```python
from build123d import *

# Parameters (mm, degrees)
SKETCH1_W           = 75
SKETCH1_H           = 90
BOSS_EXTRUDE1_DEPTH = 50
SKETCH2_W           = 75
SKETCH2_H           = 90
BOSS_EXTRUDE2_DEPTH = 10
BOSS_EXTRUDE2_TAPER = 45
SKETCH3_R           = 25
BOSS_EXTRUDE3_DEPTH = 10
SKETCH4_R           = 22.5
BOSS_EXTRUDE4_DEPTH = 30
SKETCH5_R           = 2.5
CUT_EXTRUDE1_DEPTH  = 5
CIRPATTERN1_COUNT   = 10
SKETCH6_W           = 20
SKETCH6_H           = 24
BOSS_EXTRUDE5_DEPTH = 100
SKETCH7_R           = 22.5
BOSS_EXTRUDE6_DEPTH = 10
SKETCH8_R           = 21.5
BOSS_EXTRUDE7_DEPTH = 20
SKETCH9_R           = 10
CUT_EXTRUDE2_DEPTH  = 10
FILLET1_RADIUS      = 45
FILLET1_LENGTH      = 75
SKETCH10_R          = 37.5
BOSS_EXTRUDE8_DEPTH = 10
BOSS_EXTRUDE8_TAPER = 45
SKETCH11_R          = 17.5
CUT_EXTRUDE3_DEPTH  = 20
FILLET4_R           = 1
FILLET5_R           = 1


with BuildPart() as part:
    # Sketch1 → Boss-Extrude1 (new, symmetric)
    with BuildSketch(Plane.XY):
        Rectangle(SKETCH1_W, SKETCH1_H)
    extrude(amount=BOSS_EXTRUDE1_DEPTH, both=True)

    # Sketch2 → Boss-Extrude2 (add)
    with BuildSketch(Plane(origin=(0, 0, -50), x_dir=(-1, 0, 0), z_dir=(0, 0, -1))):
        Rectangle(SKETCH2_W, SKETCH2_H)
    extrude(amount=BOSS_EXTRUDE2_DEPTH, taper=BOSS_EXTRUDE2_TAPER)

    # Sketch3 → Boss-Extrude3 (add)
    with BuildSketch(Plane(origin=(0, 0, -60), x_dir=(-1, 0, 0), z_dir=(0, 0, -1))):
        Circle(SKETCH3_R)
    extrude(amount=BOSS_EXTRUDE3_DEPTH)

    # Sketch4 → Boss-Extrude4 (add)
    with BuildSketch(Plane(origin=(0, 0, -70), x_dir=(-1, 0, 0), z_dir=(0, 0, -1))):
        Circle(SKETCH4_R)
    extrude(amount=BOSS_EXTRUDE4_DEPTH)

    # Sketch5 → Cut-Extrude1 (cut)
    with BuildSketch(Plane(origin=(0, 0, -100), x_dir=(-1, 0, 0), z_dir=(0, 0, -1))):
        with Locations((18, 0)):
            Circle(SKETCH5_R)
    cut_extrude1 = extrude(amount=-CUT_EXTRUDE1_DEPTH, mode=Mode.SUBTRACT)

    # CirPattern1: Cut-Extrude1 ×10 about axis
    cirpattern1_axis = Axis((0, 0, 0), (0, 0, 1))
    for i in range(1, CIRPATTERN1_COUNT):
        add(cut_extrude1.rotate(cirpattern1_axis, i * 360 / CIRPATTERN1_COUNT), mode=Mode.SUBTRACT)

    # Sketch6 → Boss-Extrude5 (add)
    with BuildSketch(Plane(origin=(0, 0, -100), x_dir=(-1, 0, 0), z_dir=(0, 0, -1))):
        Rectangle(SKETCH6_W, SKETCH6_H)
    extrude(amount=BOSS_EXTRUDE5_DEPTH)

    # Sketch7 → Boss-Extrude6 (add)
    with BuildSketch(Plane(origin=(0, 0, -200), x_dir=(-1, 0, 0), z_dir=(0, 0, -1))):
        Circle(SKETCH7_R)
    extrude(amount=BOSS_EXTRUDE6_DEPTH)

    # Sketch8 → Boss-Extrude7 (add)
    with BuildSketch(Plane(origin=(0, 0, -210), x_dir=(-1, 0, 0), z_dir=(0, 0, -1))):
        Circle(SKETCH8_R)
    extrude(amount=BOSS_EXTRUDE7_DEPTH)

    # Sketch9 → Cut-Extrude2 (cut)
    with BuildSketch(Plane(origin=(0, 0, -230), x_dir=(-1, 0, 0), z_dir=(0, 0, -1))):
        Circle(SKETCH9_R)
    extrude(amount=-CUT_EXTRUDE2_DEPTH, mode=Mode.SUBTRACT)

    # Fillet1: full round fillet: the end face becomes a half cylinder, R = half its width
    fillet1_face = Plane((0, 0, 50), x_dir=(1, 0, 0), z_dir=(0, 0, 1))  # on the end face: x along it, z out of the body
    fillet1_slab = fillet1_face.offset(-FILLET1_RADIUS / 2) * Box(FILLET1_LENGTH, 2 * FILLET1_RADIUS, FILLET1_RADIUS, mode=Mode.PRIVATE)  # the body's end, R deep
    fillet1_round = Plane((0, 0, 5), x_dir=(0, 0, 1), z_dir=(1, 0, 0)) * Cylinder(FILLET1_RADIUS, FILLET1_LENGTH, mode=Mode.PRIVATE)  # its axis R under the face
    add(fillet1_slab - fillet1_round, mode=Mode.SUBTRACT)

    # Sketch10 → Boss-Extrude8 (add)
    with BuildSketch(Plane(origin=(37.5, 0, 0), x_dir=(0, 0, -1), z_dir=(1, 0, 0))):
        with Locations((-5, 0)):
            Circle(SKETCH10_R)
    extrude(amount=BOSS_EXTRUDE8_DEPTH, taper=BOSS_EXTRUDE8_TAPER)

    # Sketch11 → Cut-Extrude3 (cut)
    with BuildSketch(Plane(origin=(47.5, 0, 0), x_dir=(0, 0, -1), z_dir=(1, 0, 0))):
        with Locations(Location((-5, 0, 0), (0, 0, 90))):
            Circle(SKETCH11_R)
    extrude(amount=-CUT_EXTRUDE3_DEPTH, mode=Mode.SUBTRACT)

    # Fillet4
    fillet4_edges = [part.edges().sort_by_distance(p)[0] for p in [
        (25, 0, -60),
    ]]
    fillet(fillet4_edges, radius=FILLET4_R)

    # Fillet5
    fillet5_edges = [part.edges().sort_by_distance(p)[0] for p in [
        (-10, 0, -100),
        (-10, -12, -150),
        (0, 12, -100),
        (-10, 12, -150),
        (10, 0, -100),
        (10, 12, -150),
        (0, -12, -100),
        (10, -12, -150),
        (-10, 0, -200),
        (0, 12, -200),
        (10, 0, -200),
        (0, -12, -200),
    ]]
    fillet(fillet5_edges, radius=FILLET5_R)


solid = part.part
```
Verification items for the finished model (mm, model axes). A direction names the side the tool comes from. Round coordinates to 2 decimals unless told otherwise and drop trailing zeros. Write each loop counter-clockwise with the first axis right and the second up, starting at its lowest first coordinate (ties: lowest second). Pieces come first, ordered by that corner, then holes. Notation, with made-up numbers: (-11.5, 73.5) -> (44.5, 73.5) arc R27 ccw to (44.5, 99.5) -> close; hole circle Ø4 at (30.5, 0.25). An arc over 180 degrees is marked (long way). Write each question's results on one line, items separated by ' | '. Start each with the question number.
1. Cross-section at A-A (z = -174.5). Enter the section's corners in (x, y).
2. Depth check by flat-ended pin: P1, Ø4, axis at y = 6, z = -180, coming from the -X side; P2, Ø8, axis at x = 9, z = -186.5, coming from the -Y side; P3, Ø1, axis at x = -19, y = 13.5, coming from the +Z side. Enter the tip coordinate at first touch or a pass-through.
3. Cross-section at C-C (z = -76.5). Enter the section's corners in (x, y), then the cut area to 3 significant figures.
4. Material ranges on probe 1 along X at (y, z) = (31, 37); probe 2 along Z at (x, y) = (41.5, -7); probe 3 along Z at (x, y) = (8, -15.5), recorded low to high. Write a range as from..to.
5. Draft check along X on faces 1 (the flat face through (10, 0, -149)), 2 (the cylindrical face through (4.9, 14.71, -97.54)), 3 (the flat face through (0, 12, -149)), 4 (the flat face through (15, -11, -95)). Enter one of: +X half, -X half, draft (parallel to the pull), parting line (faces both ways), or undercut.
6. Cross-section at B-B (x = 41.5). Enter the section's corners in (y, z).
7. Set-up check for faces 5 (the flat face through (0, -15, -100)), 6 (the cylindrical face through (-10.382, -19.961, -84.79)), 7 (the cylindrical face through (37.64, -13.887, -5.648)): record each of +Z, -Z, +X, -X, +Y, -Y from which the full face is reachable in a straight line by a thin tool's end or side.
Solutions:
1) outline: (-10, -11) arc R1 ccw to (-9, -12) -> (9, -12) arc R1 ccw to (10, -11) -> (10, 11) arc R1 ccw to (9, 12) -> (-9, 12) arc R1 ccw to (-10, 11) -> close
2) P1: stops at x = -10 | P2: stops at y = -12 | P3: stops at z = 48.08
3) outline: circle Ø45 at (0, 0) | area: 1,590 mm2
4) probe 1: x = -37.5..37.5 | probe 2: z = -27.76..-11.04, 21.04..37.76 | probe 3: z = -230..-200, -100..47.25
5) face 1: +X half | face 2: undercut | face 3: draft | face 4: undercut
6) outline: circle Ø67 at (0, 5); hole circle Ø35 at (0, 5)
7) face 5: none | face 6: -Z | face 7: +X
